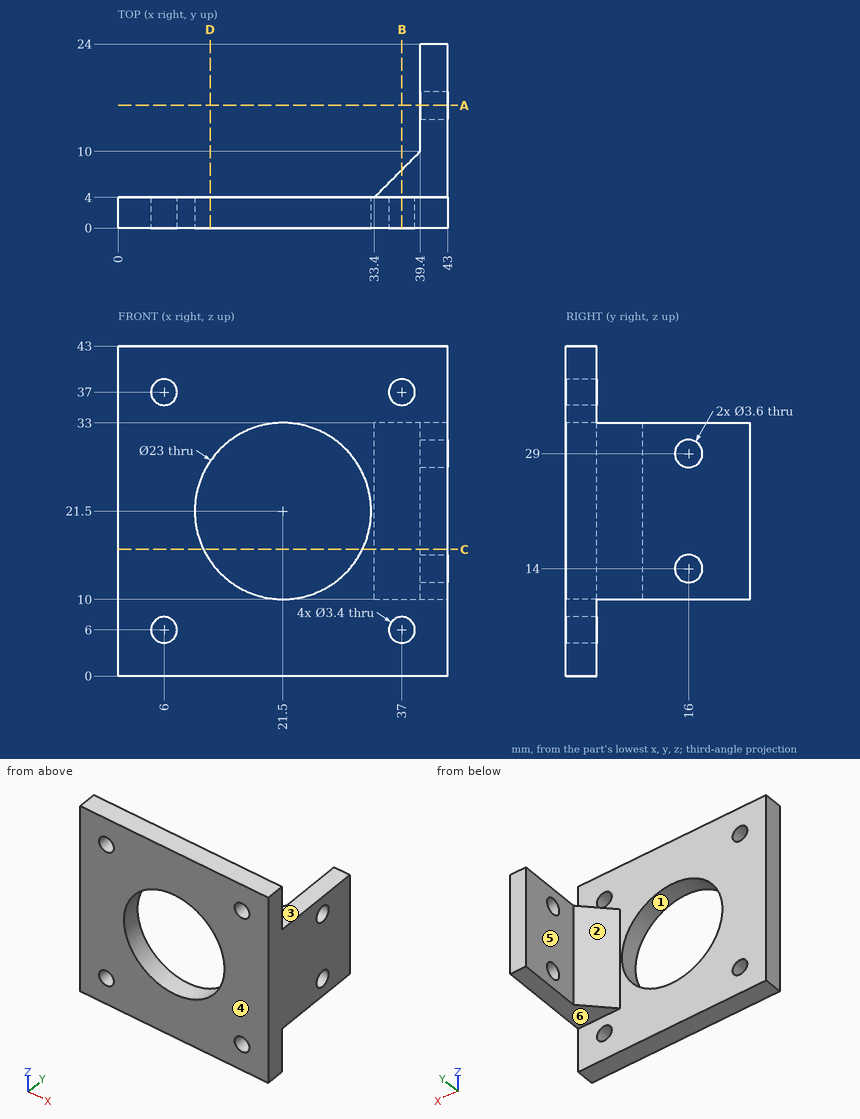
Input: dimensioned drawing with shaded views. Units: mm. Origin: part minimum x, y, z. A direction names the side the tool comes from. Give positions to 0.01 mm unless a question says otherwise; leave off trailing zeros. Loops run counter-clockwise (first coordinate to the right, second up) from the corner with the lowest first, then second, coordinate; pieces in that order, holes last. Notation, with made-up numbers: (57.25, 32) - (80.25, 32) arc R31 ccw to (80.25, 58) - close; hole circle Ø11 at (54.5, -30.5). An arc over 180 degrees is marked (long way). Answer as CSV lines item,"result". Start each with the question number.
(1) Reachability of the marked faces 4, 5 and 6 from +Z, -Z, +X, -X, +Y, -Y: full face, straight path, thin tool, end or side. Return the list, or none.
(2) Section query C-C (z = 16.5). Output: boundary loops of the cut face in (x, y).
(3) Section query B-B (x = 37). Output: boundary loops of the cut face in (y, z), and give its area (3 significant figures).
(4) Mould query, pull axis X, two halves, no side actions, for the marked faces 1, 2 and 3. Classes: +X half, -X half, draft (parallel to the pull), parting line (faces both ways), or undercut.
(5) Pin query (flat end, axial travel): P1, Ø3, axis at x = 6, z = 37, coming from the +Y side; P2, Ø4.5, axis at x = 37, z = 37, coming from the +Y side; P3, Ø10.5, axis at x = 37.5, y = 10, coming from the -Z side; P4, Ø11, axis at y = 13.5, z = 24, coming from the -X side. Return the tip coordinate at first contact, or that it passes through.
(6) Section query A-A (y = 16). Output: boundary loops of the cut face in (x, z).
(7) Section query D-D (x = 12). Output: boundary loops of the cut face in (y, z), and give its area (3 significant figures).
(8) Ray query, line 1 along Z through (x, y) = (6, 2.7); line 2 along Z through (x, y) = (40.7, 16); line 3 along Z through (x, y) = (41, 19.5). Return the intervals inside material, ascending. Write a range as [from, to].
Worked answers:
1,face 4,"+Z, -Z, +X, -X, -Y"
1,face 5,"+Z, -Z, -X, +Y"
1,face 6,"-Z, +X, -X, +Y"
2,outline,"(0, 0) - (11.14, 0) - (11.14, 4) - (0, 4) - close; (31.86, 0) - (43, 0) - (43, 24) - (39.4, 24) - (39.4, 10) - (33.4, 4) - (31.86, 4) - close"
3,outline,"(0, 0) - (4, 0) - (4, 4.3) - (0, 4.3) - close; (0, 7.7) - (4, 7.7) - (4, 10) - (7.6, 10) - (7.6, 33) - (4, 33) - (4, 35.3) - (0, 35.3) - close; (0, 38.7) - (4, 38.7) - (4, 43) - (0, 43) - close"
3,area,"228 mm^2"
4,face 1,"undercut"
4,face 2,"-X half"
4,face 3,"draft"
5,P1,"passes through"
5,P2,"stops at y = 4"
5,P3,"stops at z = 10"
5,P4,"stops at x = 37.4"
6,outline,"(39.4, 10) - (43, 10) - (43, 12.2) - (39.4, 12.2) - close; (39.4, 15.8) - (43, 15.8) - (43, 27.2) - (39.4, 27.2) - close; (39.4, 30.8) - (43, 30.8) - (43, 33) - (39.4, 33) - close"
7,outline,"(0, 0) - (4, 0) - (4, 15.02) - (0, 15.02) - close; (0, 27.98) - (4, 27.98) - (4, 43) - (0, 43) - close"
7,area,"120 mm^2"
8,line 1,"z = [0, 4.3], [7.7, 35.3], [38.7, 43]"
8,line 2,"z = [10, 12.2], [15.8, 27.2], [30.8, 33]"
8,line 3,"z = [10, 33]"
